```python
from build123d import *

# Parameters (mm, degrees)
SKETCH1_R                = 2.5
SKETCH1_R_2              = 1.5
BOSS_EXTRUDE1_DEPTH      = 4
SKETCH2_W                = 2.7
SKETCH2_H                = 3.154184917
CUT_EXTRUDE1_DEPTH       = 6.338539126
CUT_EXTRUDE2_DEPTH       = 9.860022573
BOSS_EXTRUDE2_REACH      = 13.474
BOSS_EXTRUDE2_END_RADIUS = 2.5
SKETCH5_R                = 1.125
BOSS_EXTRUDE3_REACH      = 18.274
BOSS_EXTRUDE3_END_RADIUS = 2.5
BOSS_EXTRUDE3_START      = -4.8
SKETCH6_R                = 1.375
CUT_EXTRUDE3_REACH       = 14.991
CUT_EXTRUDE3_END_RADIUS  = 2.5


with BuildPart() as part:
    # Sketch1 → Boss-Extrude1 (new body)
    with BuildSketch(Plane(origin=(0, 0, 0), x_dir=(1, 0, 0), z_dir=(0, 1, 0))):
        with Locations(Location((0, 0, 0), (0, 0, 270))):
            Circle(SKETCH1_R)
        with Locations(Location((0, 0, 0), (0, 0, 270))):
            Circle(SKETCH1_R_2, mode=Mode.SUBTRACT)
    extrude(amount=BOSS_EXTRUDE1_DEPTH)

    # Sketch2 → Cut-Extrude1 (cut, through all)
    with BuildSketch(Plane(origin=(0, 4, 0), x_dir=(1, 0, 0), z_dir=(0, 1, 0))):
        with Locations((0, -1.577092459)):
            Rectangle(SKETCH2_W, SKETCH2_H)
    extrude(amount=-CUT_EXTRUDE1_DEPTH, mode=Mode.SUBTRACT)

    # Sketch3 → Cut-Extrude2 (cut, through all)
    with BuildSketch(Plane(origin=(5, 0, 0), x_dir=(0, 0, -1), z_dir=(1, 0, 0))):
        with BuildLine():
            Line((-2.104162541, 2.3), (-2.104162541, 0))
            Line((-2.104162541, 0), (0.5, 0))
            ThreePointArc((0.5, 0), (-1.237214908, 0.657322297), (-2.104162541, 2.3))
        make_face()
    extrude(amount=-CUT_EXTRUDE2_DEPTH, mode=Mode.SUBTRACT)

    # Boss-Extrude2: up to this cylinder (the profile starts outside it)
    boss_extrude2_end = Plane(origin=(0, -0.152914, 0), z_dir=(0, -1, 0)) * Cylinder(BOSS_EXTRUDE2_END_RADIUS, 32.948, mode=Mode.PRIVATE)
    # Sketch5 → Boss-Extrude2 (add, up to the surface)
    with BuildSketch(Plane(origin=(0, -0.152914271, -8.295554958), x_dir=(-1, 0, 0), z_dir=(0, -0.2588190451025248, -0.9659258262890673)), mode=Mode.PRIVATE) as boss_extrude2_sk1:
        with Locations(Location((0, 0, 0), (0, 0, 90))):
            Circle(SKETCH5_R)
    boss_extrude2_tool1 = extrude(boss_extrude2_sk1.sketch, amount=-BOSS_EXTRUDE2_REACH, mode=Mode.PRIVATE) - boss_extrude2_end
    add(boss_extrude2_tool1.solids().sort_by_distance((0, -0.152914, -8.295555))[0])

    # Boss-Extrude3: up to this cylinder (the profile starts outside it)
    boss_extrude3_end = Plane(origin=(0, 1.089417, 0), z_dir=(0, -1, 0)) * Cylinder(BOSS_EXTRUDE3_END_RADIUS, 42.548, mode=Mode.PRIVATE)
    # Sketch6 → Boss-Extrude3 (add, up to the surface)
    with BuildSketch(Plane(origin=(0, -0.152914271, -8.295554958), x_dir=(-1, 0, 0), z_dir=(0, -0.2588190451025248, -0.9659258262890673)).offset(BOSS_EXTRUDE3_START), mode=Mode.PRIVATE) as boss_extrude3_sk1:
        with Locations(Location((0, 0, 0), (0, 0, 90))):
            Circle(SKETCH6_R)
    boss_extrude3_tool1 = extrude(boss_extrude3_sk1.sketch, amount=-BOSS_EXTRUDE3_REACH, mode=Mode.PRIVATE) - boss_extrude3_end
    add(boss_extrude3_tool1.solids().sort_by_distance((0, 1.089417, -3.659111))[0])

    # Cut-Extrude3: up to this cylinder (the profile starts outside it)
    cut_extrude3_end = Plane(origin=(0, 3.059919, 0), z_dir=(0, -1, 0)) * Cylinder(CUT_EXTRUDE3_END_RADIUS, 35.982, mode=Mode.PRIVATE)
    # Sketch7 → Cut-Extrude3 (cut, up to the surface)
    with BuildSketch(Plane.XY.offset(-10), mode=Mode.PRIVATE) as cut_extrude3_sk1:
        Polygon((0, 4.019838564), (-2.13014509, 4.019838564), (-2.13014509, 2.1), (2.0800272, 2.1), (2.0800272, 4.019838564), align=None)
    cut_extrude3_tool1 = extrude(cut_extrude3_sk1.sketch, amount=CUT_EXTRUDE3_REACH, mode=Mode.PRIVATE) - cut_extrude3_end
    add(cut_extrude3_tool1.solids().sort_by_distance((-0.025059, 3.059919, -10))[0], mode=Mode.SUBTRACT)


solid = part.part
```
Geometry: final body of the model. Coordinates: model frame, mm. A direction names the side the tool comes from. Coordinates: 2 decimals unless noted, no trailing zeros. Order: outer loops, then holes, each group sorted by start corner. A loop starts at its lowest first (then second) coordinate and runs counter-clockwise, first axis right, second up. Notation, with made-up numbers: (69.5, 82) -> (79.5, 82) arc R26 ccw to (79.5, 99) -> close; hole circle Ø3 at (56.25, 59.25). An arc over 180 degrees is marked (long way). Write item = value, one per line.
(1) Pin query (flat end, axial travel): pin 1 Ø1.5 at (x, y) = (-1.5, -0.5) entering from -Z; pin 2 Ø1 at (x, z) = (0, -6) entering from -Y; pin 3 Ø1.2 at (y, z) = (3, 1.5) entering from +X; pin 4 Ø1.8 at (x, z) = (0, 0) entering from -Y. Return the tip coordinate at first contact, or that it passes through.
Solved:
pin_1 = -8.37
pin_2 = -0.84
pin_3 = 2.33
pin_4 = through
(2) Line query: line 1 (X direction, y = 1.45, z = 0); line 2 (Y direction, x = -1.3, z = -2); line 3 (Z direction, x = 0, y = 3.1). Output: solid intervals per line, ascending.
Solved:
line_1 = -2.5 to -1.5, 1.5 to 2.5
line_2 = 0 to 4
line_3 = -2.5 to -1.5
(3) Access query for faces 4 (the flat face through (0, 4, -2)), 5 (the flat face through (1.35, 3, 1)). Directions: +Z, -Z, +X, -X, +Y, -Y. A direction counts if a zero-diameter tool reaches every point of the face in a straight line with its end or side. Return the directions, or none.
Solved:
face_4 = +Z, -Z, +X, -X, +Y
face_5 = +Z, +Y, -Y
(4) Pull-direction query (X, two-part tool) for faces 1 (the flat face through (0, 0, -2)), 2 (the cylindrical face through (0.1, 2.4, -2.5)), 3 (the flat face through (-1.35, 3, 1)); classes: pulls with the +X half, pulls with the -X half, needs draft (parallel to the pull), parting line crosses it, or undercut.
Solved:
face_1 = needs draft
face_2 = parting line crosses it
face_3 = undercut
(5) Cut plane D-D on x = 2.1. Return loops of the section in (y, z).
Solved:
outline = (0, -1.36) -> (4, -1.36) -> (4, 1.36) -> (0.77, 1.36) arc R2.62 ccw to (0, -0.5) -> close
(6) Cut plane A-A on z = -0.25. Return loops of the section in (x, y), plus the area to 3 significant figures.
Solved:
outline = (-2.49, 0.01) -> (-1.48, 0.01) -> (-1.48, 4) -> (-2.49, 4) -> close; (1.48, 0.01) -> (2.49, 0.01) -> (2.49, 4) -> (1.48, 4) -> close
area = 8.04 mm²
(7) Cut plane C-C on y = 2.95. Return loops of the section in (x, z).
Solved:
outline = (-1.35, 0.65) -> (-1.35, 2.1) arc R2.5 ccw (long way) to (1.35, 2.1) -> (1.35, 0.65) arc R1.5 cw (long way) to start
